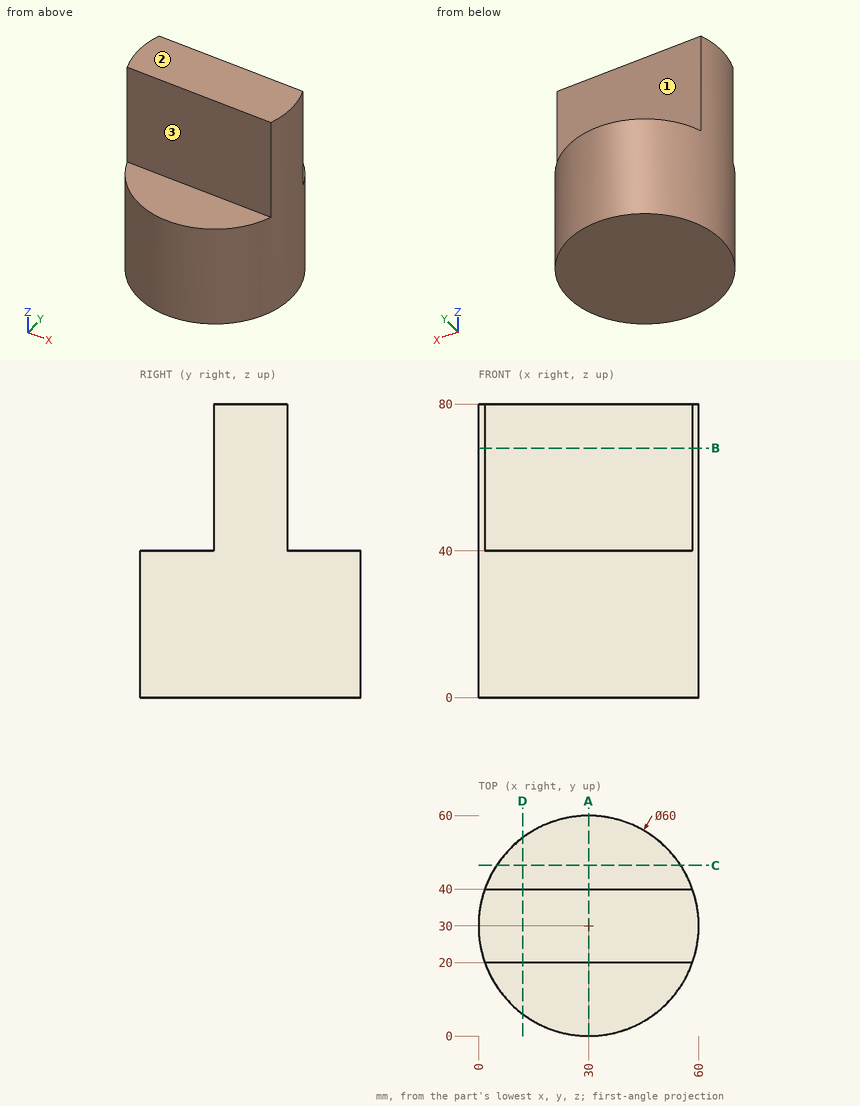
Verification items for this drawing (mm, ordinates from the low corner). A direction names the side the tool comes from. Give positions to 0.01 mm unless a question says otherwise; leave off trailing zeros. Loops run counter-clockwise (first coordinate to the right, second up) from the corner with the lowest first, then second, coordinate; pieces in that order, holes last. Notation, with made-up numbers: M 49.25,84 L 71.25,84 A30 ccw 71.25,121 Z; hole C 35.5,64.25 d1. An arc over 180 degrees is marked long. Answer as a JSON object with one key per item and string values. Group by question number.
Item 1: Material ranges on L1, parallel to Y at x = 15, z = 76; L2, parallel to Z at x = 20.5, y = 55.5; L3, parallel to Y at x = 22, z = 3, recorded low to high.
Item 2: Sectioned sample at A-A on x = 30. Record the boundary of the cut face in (y, z).
Item 3: Access from +Z, -Z, +X, -X, +Y, -Y to the whole of each face (thin tool, end or side, straight path). Record for the marked faces 1, 2 and 3.
Item 4: Gauge pin test, flat ends, axial feed: pin 1 (20 mm diameter, centred on x = 34.5, z = 63, fed in from +Y); pin 2 (3 mm diameter, centred on x = 9, z = 72, fed in from -Y); pin 3 (10 mm diameter, centred on x = 19, y = 47.5, fed in from +Z). Record the tip position at first contact, or that the pin passes through.
Item 5: Sectioned sample at D-D on x = 12. Record the boundary of the cut face in (y, z).
Item 6: Sectioned sample at B-B on z = 68. Record the boundary of the cut face in (x, y).
Item 7: Sectioned sample at C-C on y = 46.5. Record the boundary of the cut face in (x, z).
Findings below:
{
 "1": {"L1": "20 to 40", "L2": "0 to 40", "L3": "1.09 to 58.91"},
 "2": {"outline": "M 0,0 L 60,0 L 60,40 L 40,40 L 40,80 L 20,80 L 20,40 L 0,40 Z"},
 "3": {"face 1": "+Z, +X, -X, +Y", "face 2": "+Z, +X, -X, +Y, -Y", "face 3": "+Z, +X, -X, -Y"},
 "4": {"pin 1": "y = 40", "pin 2": "y = 20", "pin 3": "z = 40"},
 "5": {"outline": "M 6,0 L 54,0 L 54,40 L 40,40 L 40,80 L 20,80 L 20,40 L 6,40 Z"},
 "6": {"outline": "M 1.72,20 L 58.28,20 A30 ccw 58.28,40 L 1.72,40 A30 ccw Z"},
 "7": {"outline": "M 4.95,0 L 55.05,0 L 55.05,40 L 4.95,40 Z"}
}
